Job drawing, mm, ordinate dimensions from the low corner. One solid piece. A direction names the side the tool comes from. Coordinates: 2 decimals unless noted, no trailing zeros. Order: outer loops, then holes, each group sorted by start corner. A loop starts at its lowest first (then second) coordinate and runs counter-clockwise, first axis right, second up. Notation, with made-up numbers: (-3.75, 45) -> (36.25, 45) arc R19 ccw to (36.25, 61) -> close; hole circle Ø9 at (32, -3.5). An arc over 180 degrees is marked (long way). Use CSV: the item, a comma, the result in double quotes. Start each with the question number.
(1) Cut at A-A on x = 5. Write the cut outline in (y, z), plus the area to 3 significant figures.
(2) Cut at C-C on y = 54.5. Write the cut outline in (x, z).
(3) Pull direction Z, two halves, no side cores. Call the marked faces 1, 2, 3 and 4: pulls with the +Z half, pulls with the -Z half, needs draft (parallel to the pull), parting line crosses it, or undercut.
(4) Cut at B-B on z = 5. Write the cut outline in (x, y).
(5) Tool access for the marked faces 5 and 6: list every direction of +Z, -Z, +X, -X, +Y, -Y with a clear straight run to the whole face (end or side of a thin tool).
(6) Cut at D-D on z = 9. Write the cut outline in (x, y).
(7) Pin check, flat tips, straight feed: pin 1 Ø4 at (x, y) = (5, 55) entering from +Z; pin 2 Ø1.5 at (x, z) = (4.5, 4.5) entering from +Y; pin 3 Ø6 at (x, y) = (2, 41.5) entering from -Z; pin 4 Ø4 at (y, z) = (8.5, 3.5) entering from +X. Stop position of each tip, or through.
(8) Probe L1, parallel to Y at x = 5, z = 8.4; L2, parallel to X at y = 55, z = 8.95; L3, parallel to Z at x = 8.25, y = 56.5. List the from-to ranges inside material, lowest first.
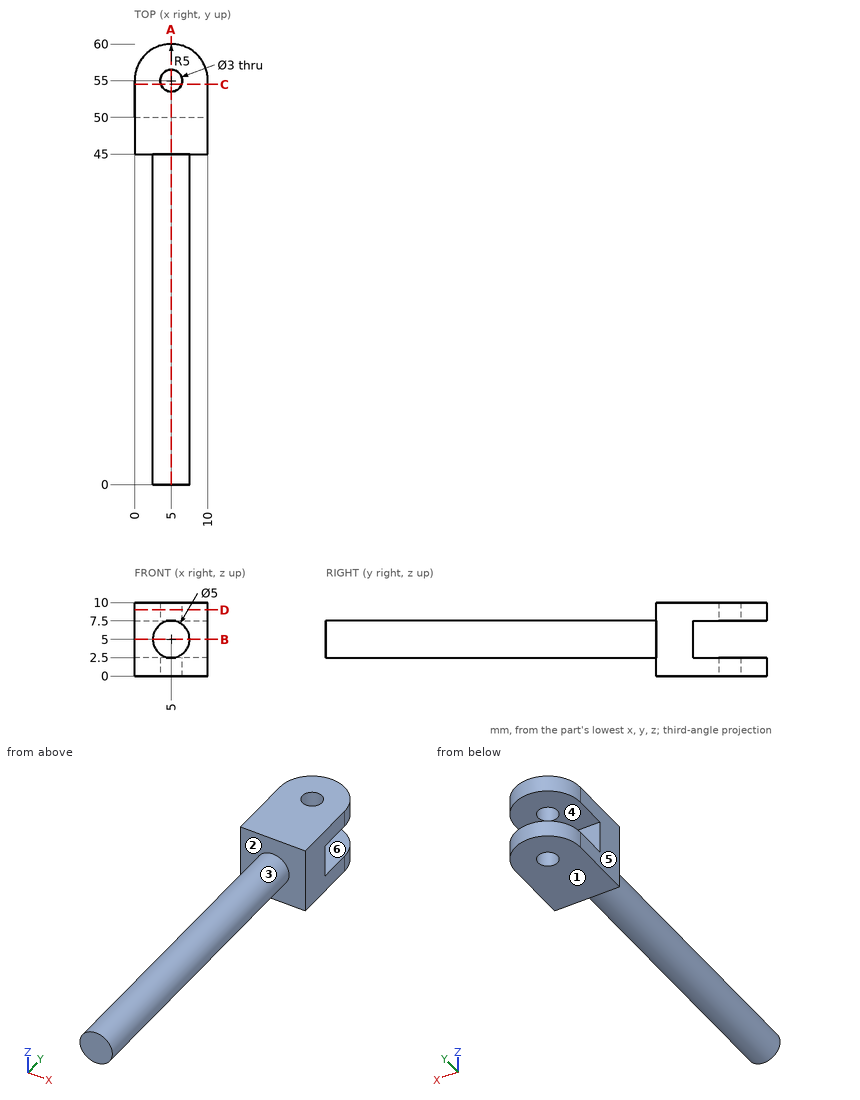
Outcome:
1,outline,"(0, 2.5) -> (45, 2.5) -> (45, 0) -> (53.5, 0) -> (53.5, 2.5) -> (50, 2.5) -> (50, 7.5) -> (53.5, 7.5) -> (53.5, 10) -> (45, 10) -> (45, 7.5) -> (0, 7.5) -> close; (56.5, 0) -> (60, 0) -> (60, 2.5) -> (56.5, 2.5) -> close; (56.5, 7.5) -> (60, 7.5) -> (60, 10) -> (56.5, 10) -> close"
1,area,"310 mm2"
2,outline,"(0, 0) -> (3.59, 0) -> (3.59, 2.5) -> (0, 2.5) -> close; (0, 7.5) -> (3.59, 7.5) -> (3.59, 10) -> (0, 10) -> close; (6.41, 0) -> (10, 0) -> (10, 2.5) -> (6.41, 2.5) -> close; (6.41, 7.5) -> (10, 7.5) -> (10, 10) -> (6.41, 10) -> close"
3,face 1,"pulls with the -Z half"
3,face 2,"needs draft"
3,face 3,"parting line crosses it"
3,face 4,"undercut"
4,outline,"(0, 45) -> (2.5, 45) -> (2.5, 0) -> (7.5, 0) -> (7.5, 45) -> (10, 45) -> (10, 50) -> (0, 50) -> close"
5,face 5,"+Z, -Z, -X, +Y, -Y"
5,face 6,"+X, -X, +Y"
6,outline,"(0, 45) -> (10, 45) -> (10, 55) arc R5 ccw to (0, 55) -> close; hole circle Ø3 at (5, 55)"
7,pin 1,"z = 10"
7,pin 2,"y = 50"
7,pin 3,"z = 2.5"
7,pin 4,"x = 7.5"
8,L1,"45 to 53.5, 56.5 to 60"
8,L2,"0 to 3.5, 6.5 to 10"
8,L3,"0 to 2.5, 7.5 to 10"
